Answer from the drawing. Dimensions are ordinates in mm from the lowest x, y and z of the part. Give positions to 0.01 mm unless a question says otherwise; leave off trailing zeros. Order: outer loops, then holes, each group sorted by start corner. A loop starts at its lowest first (then second) coordinate and runs counter-clockwise, first axis right, second up.
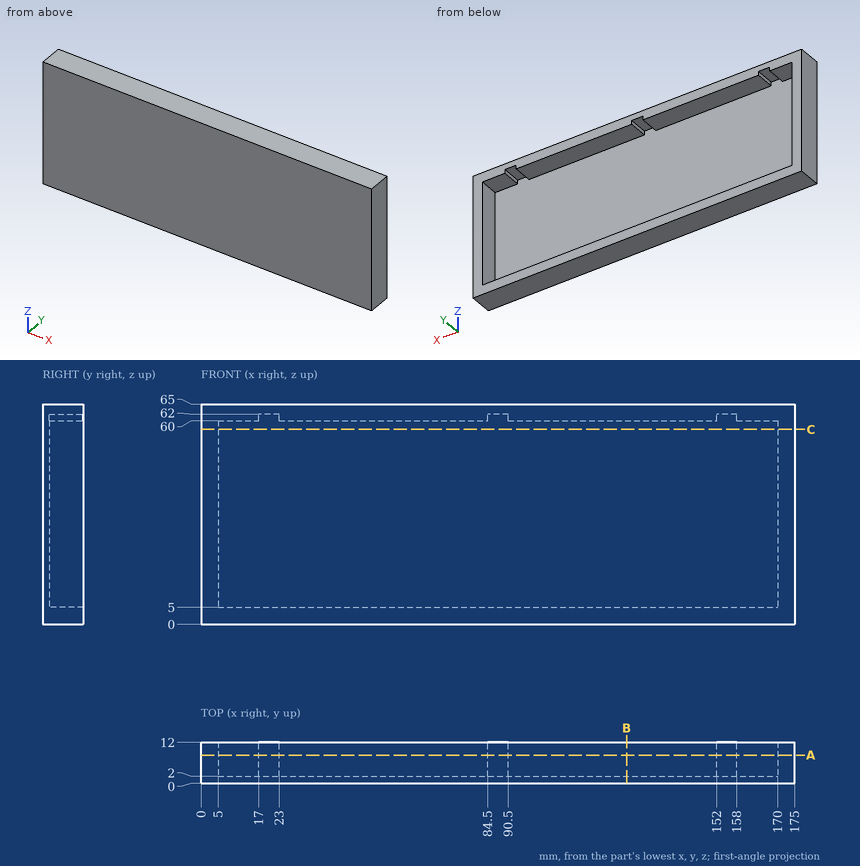
1) The part is cut by section A-A on y = 8.25. Determine the outline of the cut face in (x, z), and give its area (3 significant figures).
Final values:
outline: (0, 0) - (175, 0) - (175, 65) - (0, 65) - close; hole (5, 5) - (170, 5) - (170, 60) - (158, 60) - (158, 62) - (152, 62) - (152, 60) - (90.5, 60) - (90.5, 62) - (84.5, 62) - (84.5, 60) - (23, 60) - (23, 62) - (17, 62) - (17, 60) - (5, 60) - close
area: 2,260 mm2
2) Given pin 1 (2 mm diameter, centred on x = 89, z = 27, fed in from +Y), flat-ended and moving along its own axis, determine where the tip first touches the part or whether it passes through.
Final values:
pin 1: stops at y = 2
3) The part is cut by section B-B on x = 125.5. Determine the outline of the cut face in (y, z), and give its area (3 significant figures).
Final values:
outline: (0, 0) - (12, 0) - (12, 5) - (2, 5) - (2, 60) - (12, 60) - (12, 65) - (0, 65) - close
area: 230 mm2
4) The part is cut by section C-C on z = 57.5. Determine the outline of the cut face in (x, y), and give its area (3 significant figures).
Final values:
outline: (0, 0) - (175, 0) - (175, 12) - (170, 12) - (170, 2) - (5, 2) - (5, 12) - (0, 12) - close
area: 450 mm2
5) Consider L1, parallel to Z at x = 82, y = 10.75; L2, parallel to Z at x = 87, y = 10.5; L3, parallel to X at y = 3.5, z = 45.5. Determine where each line is inside the solid, lowest interval first.
Final values:
L1: z = 0 to 5, 60 to 65
L2: z = 0 to 5, 62 to 65
L3: x = 0 to 5, 170 to 175
